```python
from build123d import *

# Parameters (mm, degrees)
BOSS_EXTRUDE1_DEPTH = 3.175
SKETCH2_R           = 1.2925
SKETCH2_W           = 2
SKETCH2_H           = 12
SKETCH2_W_2         = 2.75
SKETCH2_H_2         = 5
CUT_EXTRUDE1_DEPTH  = 172.061595414
FILLET1_R           = 2


with BuildPart() as part:
    # Sketch1 → Boss-Extrude1 (new body)
    with BuildSketch(Plane.XY):
        with BuildLine():
            Line((150, 7.5), (5, 11.456439237))
            ThreePointArc((5, 11.456439237), (0, 12.5), (-5, 11.456439237))
            ThreePointArc((-5, 11.456439237), (-40, 18.761364576), (-75, 11.456439237))
            ThreePointArc((-75, 11.456439237), (-92.5, 0), (-75, -11.456439237))
            ThreePointArc((-75, -11.456439237), (-40, -4.151513899), (-5, -11.456439237))
            ThreePointArc((-5, -11.456439237), (0, -12.5), (5, -11.456439237))
            Line((5, -11.456439237), (150, -7.5))
            Line((150, -7.5), (170, -7.5))
            Line((170, -7.5), (170, 7.5))
            Line((170, 7.5), (150, 7.5))
        make_face()
    extrude(amount=BOSS_EXTRUDE1_DEPTH)

    # Sketch2 → Cut-Extrude1 (cut, through all)
    with BuildSketch(Plane.XY.offset(3.175)):
        with Locations((-80, 0)):
            Circle(SKETCH2_R)
        with Locations((54.666666667, 0)):
            Circle(SKETCH2_R)
        with Locations((109.333333333, 0)):
            Circle(SKETCH2_R)
        Circle(SKETCH2_R)
        with Locations((164, 0)):
            Rectangle(SKETCH2_W, SKETCH2_H)
        with Locations((151.3, 0)):
            Rectangle(SKETCH2_W_2, SKETCH2_H_2)
    extrude(amount=-CUT_EXTRUDE1_DEPTH, mode=Mode.SUBTRACT)

    # Fillet1
    fillet1_edges = [part.edges().sort_by_distance(p)[0] for p in [
        (170, 7.5, 1.5875),
        (170, -7.5, 1.5875),
        (150, -7.5, 1.5875),
        (150, 7.5, 1.5875),
    ]]
    fillet(fillet1_edges, radius=FILLET1_R)


solid = part.part
```
Geometry check sheet. Reference: the model listing, model coordinates, mm. Round coordinates to 2 decimals unless told otherwise and drop trailing zeros. Order: outer loops, then holes, each group sorted by start corner. A loop starts at its lowest first (then second) coordinate and runs counter-clockwise, first axis right, second up. Notation, with made-up numbers: (-1, 0.25) - (33, 0.25) arc R15 cw to (33, 4.25) - close; hole circle Ø2 at (85, -35.75). An arc over 180 degrees is marked (long way). Use a Markdown table: item, result. Add a question column.
1) Thickness scan on line 1 along Y through (x, z) = (-80, 2); line 2 along Y through (x, z) = (-13.5, 2.1); line 3 along Y through (x, z) = (18.5, 2.5). Record the ranges inside material, lowest first.
2) Section check B-B (x = 32.5). Record the cut outline in (y, z) (3 decimals), then the cut area to 3 significant figures.
3) Gauge pin test, flat ends, axial feed: P1, Ø1.6, axis at x = 109.33, y = 0, coming from the +Z side; P2, Ø1.6, axis at x = 155.5, z = 1.5, coming from the +Y side; P3, Ø3.5, axis at x = -80, y = 0, coming from the -Z side; P4, Ø1, axis at x = 160, z = 2, coming from the -Y side. Record the tip position at first contact, or that the pin passes through.
4) Mould release check, pull along X, two halves, no side actions. Record for faces 1 (the cylindrical face through (-92.495, 0.347, 1.565)), 2 (the flat face through (37, 0, 0)): released by +X, released by -X, zero draft, split by the parting line, or undercut.
5) Section check C-C (x = -33). Record the cut outline in (y, z) (3 decimals).
6) Section check A-A (z = 0.5). Record the cut outline in (x, y) (1 decimal), then the cut area to 3 significant figures.
Established:
| question | item | result |
|---|---|---|
| 1 | line 1 | -12.5 to -1.29, 1.29 to 12.5 |
| 1 | line 2 | -8.26 to 14.65 |
| 1 | line 3 | -11.09 to 11.09 |
| 2 | outline | (-10.706, 0) - (10.706, 0) - (10.706, 3.175) - (-10.706, 3.175) - close |
| 2 | area | 68.0 mm2 |
| 3 | P1 | through |
| 3 | P2 | y = 7.5 |
| 3 | P3 | z = 0 |
| 3 | P4 | y = -7.5 |
| 4 | face 1 | undercut |
| 4 | face 2 | zero draft |
| 5 | outline | (-4.432, 0) - (18.481, 0) - (18.481, 3.175) - (-4.432, 3.175) - close |
| 6 | outline | (-75, -11.5) arc R87.5 cw to (-5, -11.5) arc R12.5 ccw to (5, -11.5) - (150, -7.5) - (168, -7.5) arc R2 ccw to (170, -5.5) - (170, 5.5) arc R2 ccw to (168, 7.5) - (150, 7.5) - (5, 11.5) arc R12.5 ccw to (-5, 11.5) arc R87.5 ccw to (-75, 11.5) arc R12.5 ccw (long way) to start; hole circle Ø2.6 at (-80, 0); hole circle Ø2.6 at (0, 0); hole circle Ø2.6 at (54.7, 0); hole circle Ø2.6 at (109.3, 0); hole (149.9, -2.5) - (152.7, -2.5) - (152.7, 2.5) - (149.9, 2.5) - close; hole (163, -6) - (165, -6) - (165, 6) - (163, 6) - close |
| 6 | area | 5,200 mm2 |
